Autodesk Inventor part; units mm, degrees
ref_plane "YZ Plane" through (0, 0, 0) normal (1, 0, 0) x (0, 1, 0)
ref_plane "XZ Plane" through (0, 0, 0) normal (0, 1, 0) x (-1, 0, 0)
ref_plane "XY Plane" through (0, 0, 0) normal (0, 0, 1) x (1, 0, 0)
sketch "Sketch1" plane through (0, 0, 0) normal (0, 1, 0) x (-1, 0, 0)
  line L0 (97.155, 146.05) -> (-97.155, 146.05)
  line L1 (-97.155, 146.05) -> (-97.155, -146.05)
  line L2 (-97.155, -146.05) -> (97.155, -146.05)
  line L3 (97.155, -146.05) -> (97.155, 146.05)
  line L4 (97.155, 146.05) -> (-97.155, -146.05) construction
  line L5 (-97.155, 146.05) -> (97.155, -146.05) construction
  line L6 (97.155, -146.05) -> (78.105, -146.05)
  line L7 (78.105, -146.05) -> (59.055, -146.05)
  line L8 (59.055, -146.05) -> (59.055, -152.4)
  line L9 (59.055, -152.4) -> (78.105, -152.4)
  line L10 (78.105, -152.4) -> (78.105, -146.05)
  line L11 (40.005, -146.05) -> (20.955, -146.05)
  line L12 (40.005, -152.4) -> (40.005, -146.05)
  line L13 (20.955, -146.05) -> (20.955, -152.4)
  line L14 (20.955, -152.4) -> (40.005, -152.4)
  line L15 (1.905, -146.05) -> (-17.145, -146.05)
  line L16 (1.905, -152.4) -> (1.905, -146.05)
  line L17 (-17.145, -146.05) -> (-17.145, -152.4)
  line L18 (-17.145, -152.4) -> (1.905, -152.4)
  line L19 (78.105, 146.05) -> (59.055, 146.05)
  line L20 (59.055, 146.05) -> (59.055, 152.4)
  line L21 (59.055, 152.4) -> (78.105, 152.4)
  line L22 (78.105, 152.4) -> (78.105, 146.05)
  line L23 (40.005, 146.05) -> (20.955, 146.05)
  line L24 (40.005, 152.4) -> (40.005, 146.05)
  line L25 (20.955, 146.05) -> (20.955, 152.4)
  line L26 (20.955, 152.4) -> (40.005, 152.4)
  line L27 (1.905, 146.05) -> (-17.145, 146.05)
  line L28 (1.905, 152.4) -> (1.905, 146.05) construction
  line L29 (-17.145, 146.05) -> (-17.145, 152.4) construction
  line L30 (-17.145, 152.4) -> (1.905, 152.4) construction
  line L31 (-23.495, 152.4) -> (-23.495, 146.05)
  line L32 (-23.495, 146.05) -> (-42.545, 146.05)
  line L33 (-42.545, 146.05) -> (-42.545, 152.4)
  line L34 (-42.545, 152.4) -> (-23.495, 152.4)
  line L35 (-23.495, 146.05) -> (-42.545, 146.05)
  line L36 (-23.495, -152.4) -> (-23.495, -146.05)
  line L37 (-23.495, -146.05) -> (-42.545, -146.05)
  line L38 (-42.545, -146.05) -> (-42.545, -152.4)
  line L39 (-42.545, -152.4) -> (-23.495, -152.4)
  point P0 (0, 0)
  dimension "d0" = 292.1
  dimension "d1" = 194.31
  dimension "d2" = 19.05
  dimension "d3" = 19.05
  dimension "d4" = 6.35
  dimension "d7" = 38.1
  dimension "d14" = 6.35
  dimension "d15" = 19.05
extrude "Extrusion2" add sketch "Sketch1" along normal blind 6.35 contours L3 L2 L1 L0 | L0 L20 L21 L22 | L10 L9 L8 L2 | L0 L25 L26 L24 | L12 L14 L13 L2 | L0 L33 L34 L31 | L36 L39 L38 L2
properties part number "ramp"
The listing builds one solid part. Answer for the finished solid, in the listing's coordinates (mm). A direction names the side the tool comes from. Coordinates: 2 decimals unless noted, no trailing zeros. Write each loop counter-clockwise with the first axis right and the second up, starting at its lowest first coordinate (ties: lowest second). Pieces come first, ordered by that corner, then holes. Notation, with made-up numbers: M 19.5,39 L 58.5,39 A20 ccw 58.5,61 Z; hole C 36,73 d2. An arc over 180 degrees is marked long. Put each result on its own line as item: value. Start each with the question number.
1. Which of the six approach directions +Z, -Z, +X, -X, +Y, -Y give full straight-line access (tool end or side, diameter ignored) to faces 4 (the flat face through (-88, 3, 146.05)), 5 (the flat face through (-40.005, 3, 149)), 6 (the flat face through (-59.055, 3, -149))?
2. A cutting plane is placed at B-B on x = 16.5. Write down the section's boundary in (y, z).
3. Flat-ended cylindrical pins translate along their axes: P1, Ø1.9, axis at y = 4, z = 150.5, coming from the +X side (3 decimals); P2, Ø1.9, axis at y = 2.5, z = -151, coming from the -X side (3 decimals); P3, Ø1.9, axis at x = 83.5, y = 3, coming from the -Z side. Find the tip coordinate at first contact, or state that the pin passes through.
4. For a pull along X with two mould halves and no side action, classify faces 1 (the flat face through (-97.155, 3, -2)), 2 (the flat face through (-30, 3, -152.4)), 3 (the flat face through (-50, 3, 146.05)) as pulls with the +X half, pulls with the -X half, needs draft (parallel to the pull), parting line crosses it, or undercut.
5. A cutting plane is placed at A-A on y = 3. Write down the section's boundary in (x, z) (3 decimals), then the cut area to 3 significant figures.
6. Consider line 1 (Z direction, x = 10, y = 2.25). Determine where the line is inside the solid, lowest interval first. Write a range as from..to.
Resolved:
1. face 4: +Z, -X, +Y, -Y
1. face 5: +Z, +Y, -Y
1. face 6: -Z, +Y, -Y
2. outline: M 0,-146.05 L 6.35,-146.05 L 6.35,146.05 L 0,146.05 Z
3. P1: stops at x = 42.545
3. P2: stops at x = -78.105
3. P3: stops at z = -146.05
4. face 1: pulls with the -X half
4. face 2: needs draft
4. face 3: undercut
5. outline: M -97.155,-146.05 L -78.105,-146.05 L -78.105,-152.4 L -59.055,-152.4 L -59.055,-146.05 L -40.005,-146.05 L -40.005,-152.4 L -20.955,-152.4 L -20.955,-146.05 L 23.495,-146.05 L 23.495,-152.4 L 42.545,-152.4 L 42.545,-146.05 L 97.155,-146.05 L 97.155,146.05 L 42.545,146.05 L 42.545,152.4 L 23.495,152.4 L 23.495,146.05 L -20.955,146.05 L -20.955,152.4 L -40.005,152.4 L -40.005,146.05 L -59.055,146.05 L -59.055,152.4 L -78.105,152.4 L -78.105,146.05 L -97.155,146.05 Z
5. area: 57,500 mm2
6. line 1: z = -146.05..146.05
